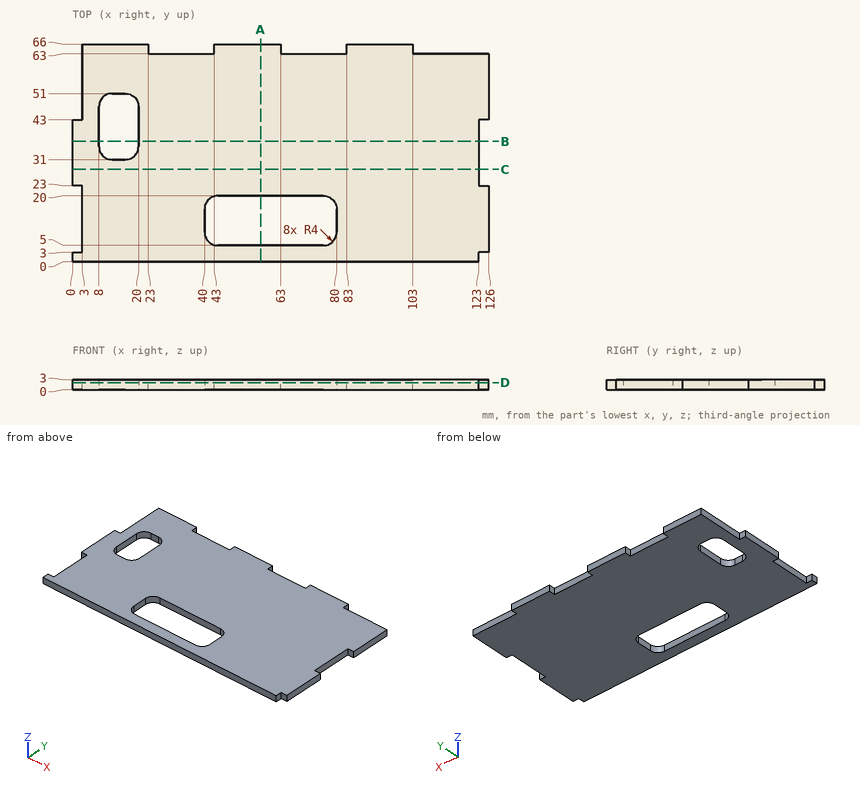
Here's the drawing with two shaded views (mm, measured from the low corner). I have some questions. Give positions to 0.01 mm unless a question says otherwise; leave off trailing zeros. Order: outer loops, then holes, each group sorted by start corner. A loop starts at its lowest first (then second) coordinate and runs counter-clockwise, first axis right, second up.
Q1. Suppose I cut it at B-B, the plane y = 36.5. Write out the boundary of the cut face in (x, z).
Q2. Suppose I cut it at D-D, the plane z = 2.2. Count the separate pieces of the cut face and the enclosed holes in it, and give its area (3 significant figures).
Q3. I'm going to push flat-ended pins straight in: P1, Ø0.9, axis at x = 124.5, z = 2, coming from the -Y side; P2, Ø1.5, axis at x = 32.5, z = 1.5, coming from the +Y side; P3, Ø1, axis at y = 59.5, z = 2, coming from the -X side. Where does each tip first touch, or does it pass through?
Q4. Suppose I cut it at C-C, the plane y = 28. Write out the boundary of the cut face in (x, z), and give its area (3 significant figures).
Q5. Suppose I cut it at A-A, the plane x = 57. Write out the boundary of the cut face in (y, z).
Q6. If I drill on line 1 along Y through (x, z) = (70.5, 1.95); line 2 along X through (y, z) = (10, 2); line 3 along X through (y, z) = (41.5, 0.4), over which ranges is the centre line in solid material (lowest first)?
Solution:
1. outline: (0, 0) - (8, 0) - (8, 3) - (0, 3) - close; (20, 0) - (123, 0) - (123, 3) - (20, 3) - close
2. separate pieces: 1
2. enclosed holes: 2
2. area: 7,120 mm2
3. P1: stops at y = 3
3. P2: stops at y = 63
3. P3: stops at x = 3
4. outline: (0, 0) - (123, 0) - (123, 3) - (0, 3) - close
4. area: 369 mm2
5. outline: (0, 0) - (5, 0) - (5, 3) - (0, 3) - close; (20, 0) - (66, 0) - (66, 3) - (20, 3) - close
6. line 1: y = 0 to 5, 20 to 63
6. line 2: x = 3 to 40, 80 to 126
6. line 3: x = 0 to 8, 20 to 123
